The drawing under review shows one solid part. Ordinate dimensions are in mm from its lowest x, y, z. A direction names the side the tool comes from. Coordinates: 2 decimals unless noted, no trailing zeros. Order: outer loops, then holes, each group sorted by start corner. A loop starts at its lowest first (then second) coordinate and runs counter-clockwise, first axis right, second up. Notation, with made-up numbers: (67.5, 44) -> (111.5, 44) arc R15 ccw to (111.5, 66) -> close; hole circle Ø1 at (-25, 19). An arc over 180 degrees is marked (long way). Use one line per item in the form item = value.
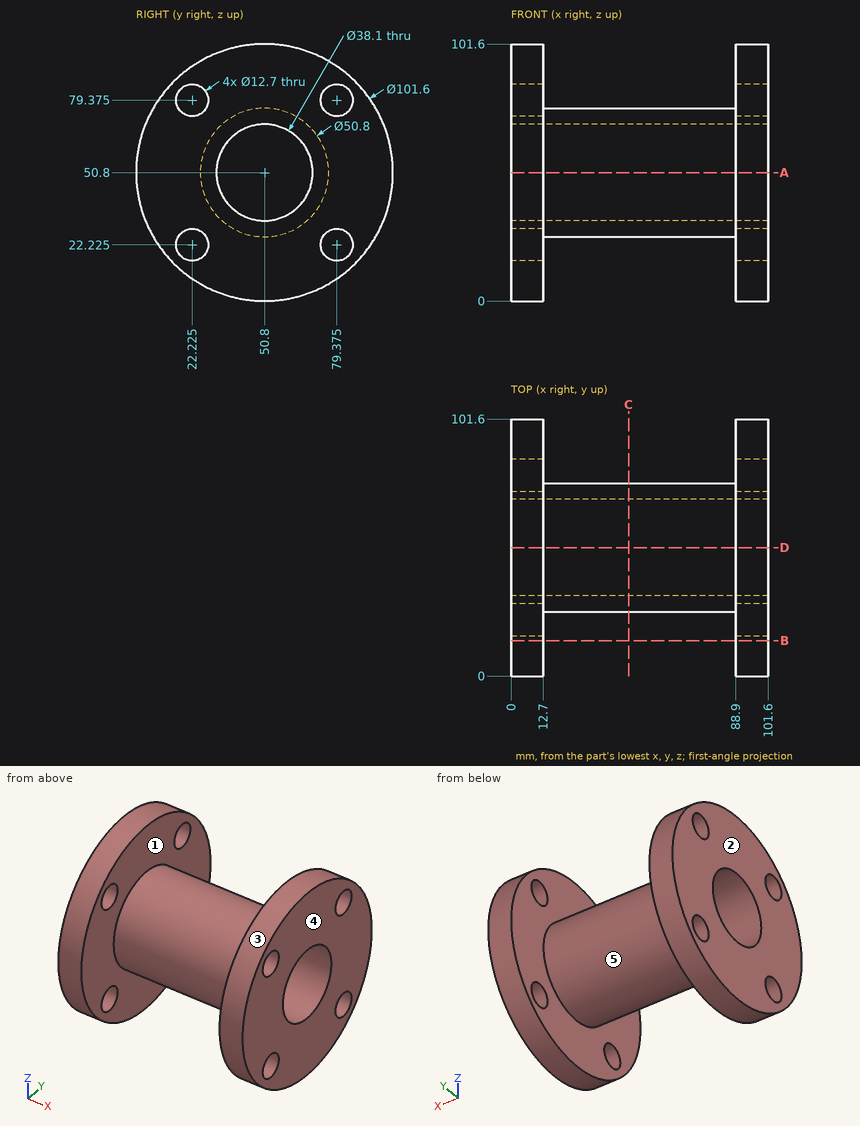
Item 1: Draft analysis for pull direction X (two halves, no side actions). For the marked faces 1, 2 and 3, state which applies: released by +X, released by -X, zero draft, split by the parting line, or undercut.
Results found:
face_1 = undercut
face_2 = released by -X
face_3 = zero draft
Item 2: We need section C-C (x = 46.5). Write out the cut boundary in (y, z).
Results found:
outline = circle Ø50.8 at (50.8, 50.8); hole circle Ø38.1 at (50.8, 50.8)
Item 3: Tool access review of the marked faces 4 and 5: name each direction out of +Z, -Z, +X, -X, +Y, -Y from which nothing blocks a thin tool from reaching the whole face with its end or side.
Results found:
face_4 = +Z, -Z, +X, +Y, -Y
face_5 = none
Item 4: To check wall thickness, follow L1, parallel to X at y = 75.5, z = 17; L2, parallel to Y at x = 9, z = 82; L3, parallel to Z at x = 93, y = 51. State the ranges of each line that lie inside material, in increasing order. Write a range as from..to.
Results found:
L1 = 0..12.7, 88.9..101.6
L2 = 10.71..16.44, 28.01..73.59, 85.16..90.89
L3 = 0..31.75, 69.85..101.6
Item 5: We need section B-B (y = 14). Write out the cut boundary in (x, z), plus the area to 3 significant figures.
Results found:
outline = (0, 15.78) -> (12.7, 15.78) -> (12.7, 85.82) -> (0, 85.82) -> close; (88.9, 15.78) -> (101.6, 15.78) -> (101.6, 85.82) -> (88.9, 85.82) -> close
area = 1,780 mm²
Item 6: We need section A-A (z = 50.8). Write out the cut boundary in (x, y).
Results found:
outline = (0, 0) -> (12.7, 0) -> (12.7, 25.4) -> (88.9, 25.4) -> (88.9, 0) -> (101.6, 0) -> (101.6, 31.75) -> (0, 31.75) -> close; (0, 69.85) -> (101.6, 69.85) -> (101.6, 101.6) -> (88.9, 101.6) -> (88.9, 76.2) -> (12.7, 76.2) -> (12.7, 101.6) -> (0, 101.6) -> close
Item 7: Clearance check with flat-ended pins moving along their axes: pin 1 (1 mm diameter, centred on x = 29, z = 35, fed in from -Y); pin 2 (1 mm diameter, centred on x = 63.5, y = 35, fed in from +Z); pin 3 (8 mm diameter, centred on x = 66, y = 57, fed in from -Z). State where each tip first meets the part, or that it passes through.
Results found:
pin_1 = 30.53
pin_2 = 71.07
pin_3 = 25.5
